```python
from build123d import *

# Parameters (mm, degrees)
SKETCH1_R               = 20
BOSS_EXTRUDE1_DEPTH     = 40
SKETCH2_W               = 30
SKETCH2_H               = 10
SKETCH2_W_2             = 10
CUT_EXTRUDE1_DEPTH      = 40
CUT_EXTRUDE1_DEPTH_BACK = 40


with BuildPart() as part:
    # Sketch1 → Boss-Extrude1 (new body)
    with BuildSketch(Plane.XY):
        Circle(SKETCH1_R)
    extrude(amount=BOSS_EXTRUDE1_DEPTH)

    # Sketch2 → Cut-Extrude1 (cut, two sides)
    with BuildSketch(Plane(origin=(0, 0, 0), x_dir=(1, 0, 0), z_dir=(0, 1, 0))) as cut_extrude1_sk:
        with Locations((-5, -35)):
            Rectangle(SKETCH2_W, SKETCH2_H)
        with Locations((-15, -5)):
            Rectangle(SKETCH2_W_2, SKETCH2_H)
    extrude(amount=CUT_EXTRUDE1_DEPTH, mode=Mode.SUBTRACT)
    extrude(cut_extrude1_sk.sketch, amount=-CUT_EXTRUDE1_DEPTH_BACK, mode=Mode.SUBTRACT)


solid = part.part
```
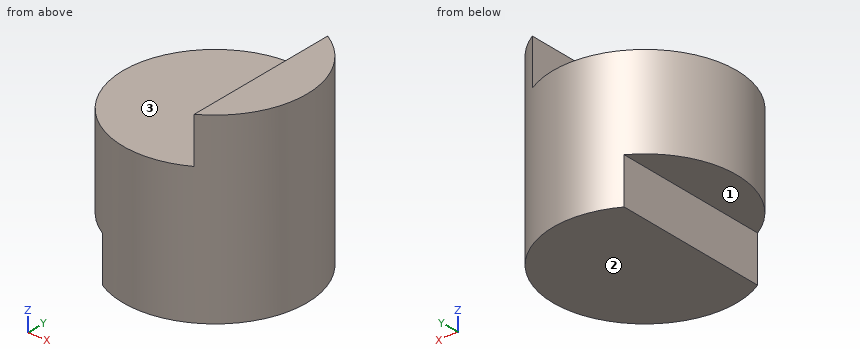
The model under review builds one solid part; all positions refer to its coordinate system, in mm. Face numbers are marked on the shaded views. A direction names the side the tool comes from. Round coordinates to 2 decimals unless told otherwise and drop trailing zeros. Loops run counter-clockwise (first coordinate to the right, second up) from the corner with the lowest first, then second, coordinate; pieces in that order, holes last. Notation, with made-up numbers: (20, 39.25) -> (61, 39.25) arc R28 ccw to (61, 59.25) -> close; hole circle Ø1 at (4.25, 63). An arc over 180 degrees is marked (long way). Answer as a JSON object with one key per item and string values. Group by question number.
1) We need section C-C on x = 0. Write out the cut boundary in (y, z), then the cut area to 3 significant figures.
2) We need section B-B on z = 17.5. Write out the cut boundary in (x, y), then the cut area to 3 significant figures.
3) For line 1 (Z direction, x = -7, y = -3.5); line 2 (Z direction, x = -14, y = -12.5); line 3 (Y direction, x = 11.5, z = 22), list the stretches that pass through material, from the lowest coordinate up. Write a range as [from, to].
4) We need section A-A on y = 10. Write out the cut boundary in (x, z).
5) For pin 1 Ø9 at (x, y) = (-12, -7.5) entering from +Z; pin 2 Ø5 at (y, z) = (-14, 25) entering from +X; pin 3 Ø3 at (x, y) = (-16.5, 6.5) entering from -Z, all flat-tipped, find the tip position at first contact; note any pin that passes through.
6) We need section D-D on y = 0. Write out the cut boundary in (x, z).
7) For the marked faces 1, 2 and 3, list the 3-axis set-ups (+Z, -Z, +X, -X, +Y, -Y) from which the entire face can be reached by the end or side of a thin tool; tool diameter is ignored.
Result set:
{
 "1": {"outline": "(-20, 0) -> (20, 0) -> (20, 30) -> (-20, 30) -> close", "area": "1,200 mm²"},
 "2": {"outline": "circle Ø40 at (0, 0)", "area": "1,260 mm²"},
 "3": {"line 1": "[0, 30]", "line 2": "[10, 30]", "line 3": "[-16.36, 16.36]"},
 "4": {"outline": "(-17.32, 10) -> (-10, 10) -> (-10, 0) -> (17.32, 0) -> (17.32, 40) -> (10, 40) -> (10, 30) -> (-17.32, 30) -> close"},
 "5": {"pin 1": "z = 30", "pin 2": "x = 16.36", "pin 3": "z = 10"},
 "6": {"outline": "(-20, 10) -> (-10, 10) -> (-10, 0) -> (20, 0) -> (20, 40) -> (10, 40) -> (10, 30) -> (-20, 30) -> close"},
 "7": {"face 1": "-Z, -X, +Y, -Y", "face 2": "-Z, +X, -X, +Y, -Y", "face 3": "+Z, -X, +Y, -Y"}
}
